Job drawing, mm, ordinate dimensions from the low corner. One solid piece. Round coordinates to 2 decimals unless told otherwise and drop trailing zeros. Write each loop counter-clockwise with the first axis right and the second up, starting at its lowest first coordinate (ties: lowest second). Pieces come first, ordered by that corner, then holes. Notation, with made-up numbers: M 1.25,-18.75 L 16.25,-18.75 A27 ccw 16.25,20.25 Z; hole C -40,-37.75 d1. An arc over 180 degrees is marked long. One line per item, written item: value. Start each with the question number.
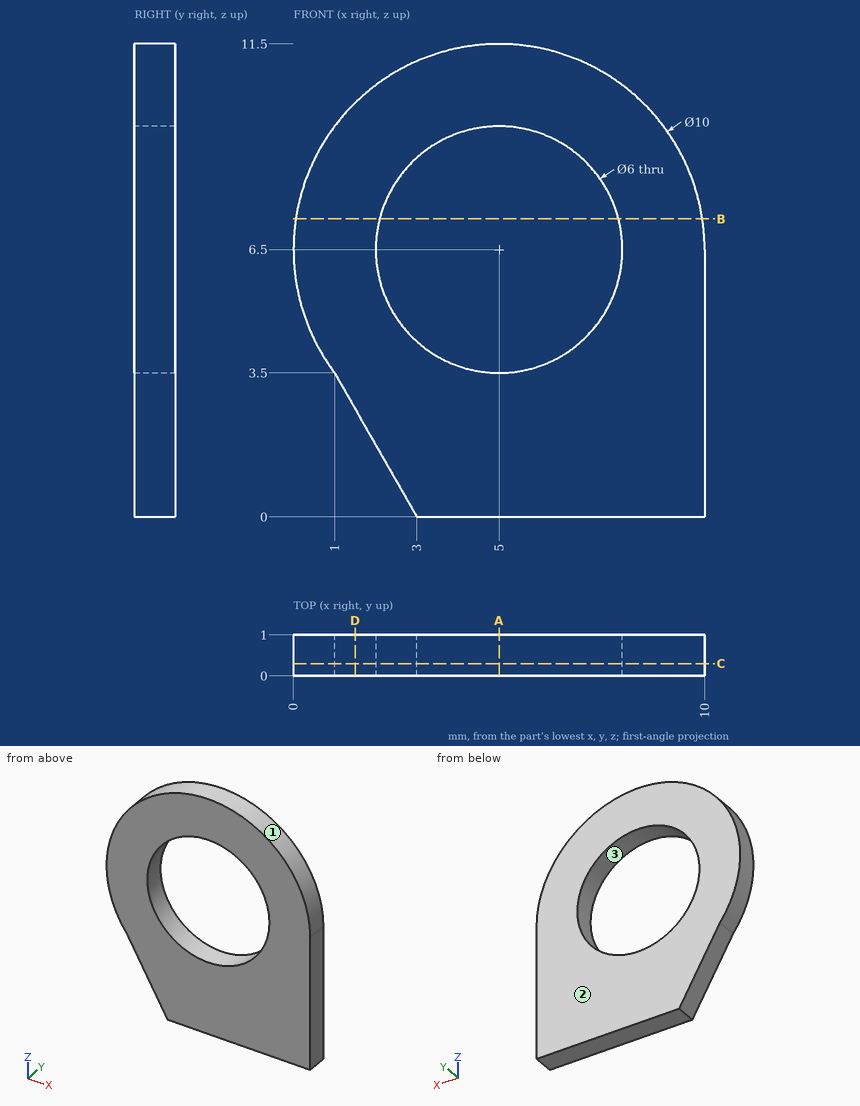
Item 1: Cut at D-D, the plane x = 1.5. Write the cut outline in (y, z) (3 decimals).
Item 2: Two-plate mould, pull along Z, no slides. Class the marked faces 1, 2 and 3: pulls with the +Z half, pulls with the -Z half, needs draft (parallel to the pull), parting line crosses it, or undercut.
Item 3: Drill centre lines: line 1 (Z direction, x = 5, y = 0.5); line 2 (X direction, y = 0.8, z = 5.5); line 3 (X direction, y = 0.75, z = 10.5). Where is each one in solid material? Low to high.
Item 4: Cut at A-A, the plane x = 5. Write the cut outline in (y, z), plus the area to 3 significant figures.
Item 5: Cut at C-C, the plane y = 0.3. Write the cut outline in (x, z).
Item 6: Drop a flat-ended pin along its axis: pin 1 (5 mm diameter, centred on x = 5, z = 6.5, fed in from +Y). Give the stop position or say it passes through.
Item 7: Cut at B-B, the plane z = 7.25. Write the cut outline in (x, y), plus the area to 3 significant figures.
Computed values:
1. outline: M 0,2.625 L 1,2.625 L 1,10.071 L 0,10.071 Z
2. face 1: parting line crosses it
2. face 2: needs draft
2. face 3: undercut
3. line 1: z = 0 to 3.5, 9.5 to 11.5
3. line 2: x = 0.1 to 2.17, 7.83 to 10
3. line 3: x = 2 to 8
4. outline: M 0,0 L 1,0 L 1,3.5 L 0,3.5 Z; M 0,9.5 L 1,9.5 L 1,11.5 L 0,11.5 Z
4. area: 5.50 mm2
5. outline: M 1,3.5 L 3,0 L 10,0 L 10,6.5 A5 ccw long Z; hole C 5,6.5 d6
6. pin 1: passes through
7. outline: M 0.06,0 L 2.1,0 L 2.1,1 L 0.06,1 Z; M 7.9,0 L 9.94,0 L 9.94,1 L 7.9,1 Z
7. area: 4.08 mm2
